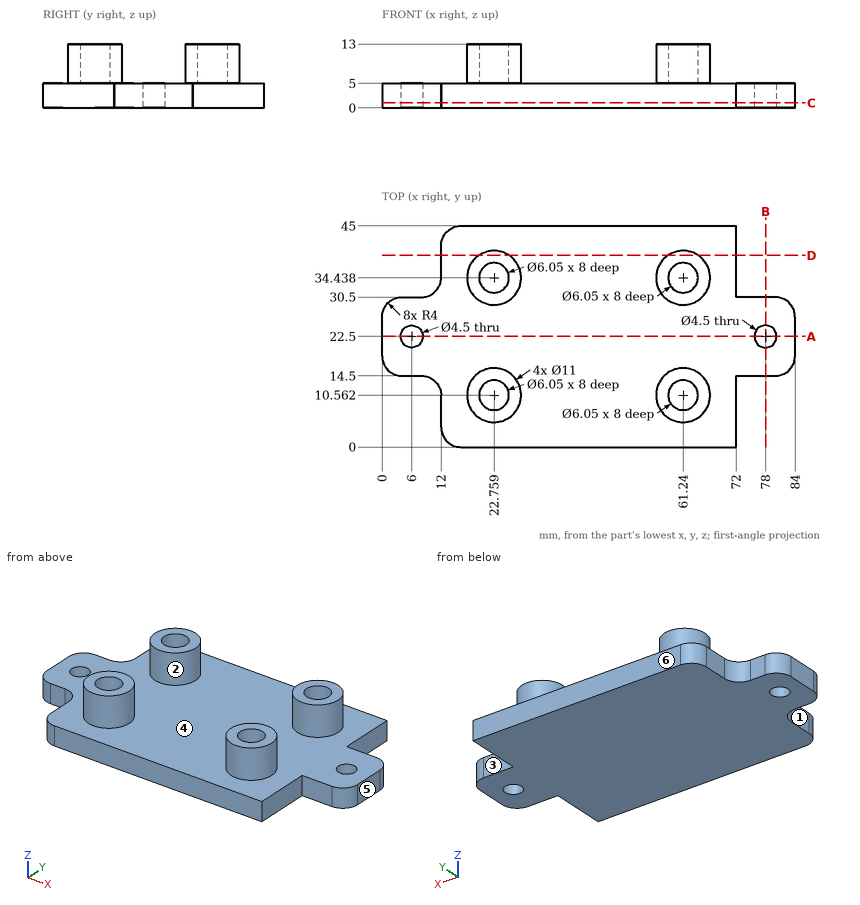
Check sheet for the drawn part. Datum: minimum x, y, z corner. Units: mm. A direction names the side the tool comes from. Round coordinates to 2 decimals unless told otherwise and drop trailing zeros. Write each loop counter-clockwise with the first axis right and the second up, starting at its lowest first coordinate (ties: lowest second). Pieces come first, ordered by that corner, then holes. Notation, with made-up numbers: (33, 31) -> (37, 31) arc R24 cw to (37, 61) -> close; hole circle Ø7 at (10.25, 59). An arc over 180 degrees is marked (long way). Write each question's results on one line, items separated by ' | '. Start each with the question number.
1. Cross-section at B-B (x = 78). Enter the section's corners in (y, z).
2. Cross-section at D-D (y = 39). Enter the section's corners in (x, z).
3. Material ranges on probe 1 along Y at (x, z) = (78, 2.5); probe 2 along X at (y, z) = (22, 2.75) (1 decimal); probe 3 along X at (y, z) = (20.5, 2) (1 decimal), recorded low to high. Write a range as from..to.
4. Cross-section at C-C (z = 1). Enter the section's corners in (x, y).
5. Cross-section at A-A (y = 22.5). Enter the section's corners in (x, z), then the cut area to 3 significant figures.
6. Depth check by flat-ended pin: P1, Ø3, axis at x = 17.5, z = 10.5, coming from the -Y side; P2, Ø3, axis at x = 60.5, y = 34.5, coming from the +Z side; P3, Ø5.5, axis at x = 77, z = 3, coming from the -Y side. Enter the tip coordinate at first touch or a pass-through.
7. Set-up check for the marked faces 1, 2 and 3: record each of +Z, -Z, +X, -X, +Y, -Y from which the full face is reachable in a straight line by a thin tool's end or side.
8. Draft check along X on the marked faces 4, 5 and 6. Enter one of: +X half, -X half, draft (parallel to the pull), parting line (faces both ways), or undercut.
Solutions:
1) outline: (14.5, 0) -> (20.25, 0) -> (20.25, 5) -> (14.5, 5) -> close; (24.75, 0) -> (30.5, 0) -> (30.5, 5) -> (24.75, 5) -> close
2) outline: (12, 0) -> (72, 0) -> (72, 5) -> (64.31, 5) -> (64.31, 13) -> (58.17, 13) -> (58.17, 5) -> (25.83, 5) -> (25.83, 13) -> (19.69, 13) -> (19.69, 5) -> (12, 5) -> close
3) probe 1: y = 14.5..20.25, 24.75..30.5 | probe 2: x = 0..3.8, 8.2..75.8, 80.2..84 | probe 3: x = 0..5, 7..77, 79..84
4) outline: (0, 18.5) arc R4 ccw to (4, 14.5) -> (8, 14.5) arc R4 cw to (12, 10.5) -> (12, 4) arc R4 ccw to (16, 0) -> (72, 0) -> (72, 14.5) -> (80, 14.5) arc R4 ccw to (84, 18.5) -> (84, 26.5) arc R4 ccw to (80, 30.5) -> (72, 30.5) -> (72, 45) -> (16, 45) arc R4 ccw to (12, 41) -> (12, 34.5) arc R4 cw to (8, 30.5) -> (4, 30.5) arc R4 ccw to (0, 26.5) -> close; hole circle Ø4.5 at (6, 22.5); hole circle Ø4.5 at (78, 22.5)
5) outline: (0, 0) -> (3.75, 0) -> (3.75, 5) -> (0, 5) -> close; (8.25, 0) -> (75.75, 0) -> (75.75, 5) -> (8.25, 5) -> close; (80.25, 0) -> (84, 0) -> (84, 5) -> (80.25, 5) -> close | area: 375 mm2
6) P1: stops at y = 6.55 | P2: stops at z = 5 | P3: stops at y = 14.5
7) face 1: +Z, -Z, -X, -Y | face 2: +Z | face 3: +Z, -Z, +X, +Y
8) face 4: undercut | face 5: +X half | face 6: draft
